Check sheet for the modelled part. Datum: model origin and axes. Units: mm. Face numbers are marked on the shaded views. A direction names the side the tool comes from. Give positions to 0.01 mm unless a question says otherwise; leave off trailing zeros. Loops run counter-clockwise (first coordinate to the right, second up) from the corner with the lowest first, then second, coordinate; pieces in that order, holes last. Notation, with made-up numbers: (12.5, 8.5) - (52.5, 8.5) arc R35 cw to (52.5, 41.5) - close; hole circle Ø10 at (-7, -14). An arc over 180 degrees is marked (long way). Use CSV: the item, a comma, the result in double quotes.
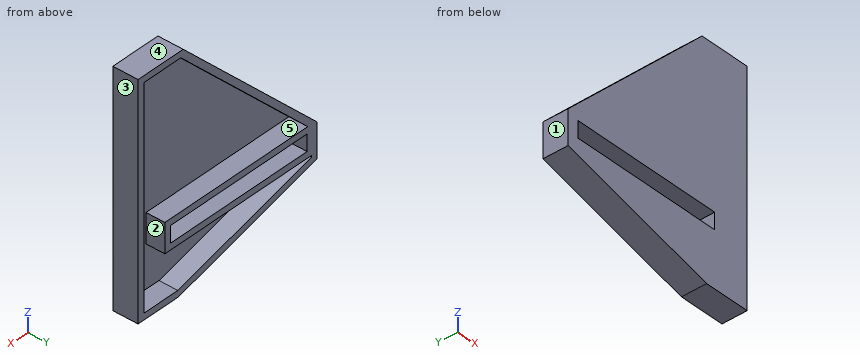
Autodesk Inventor part; units mm, degrees
ref_plane "YZ Plane" through (0, 0, 0) normal (1, 0, 0) x (0, 1, 0)
ref_plane "XZ Plane" through (0, 0, 0) normal (0, 1, 0) x (-1, 0, 0)
ref_plane "XY Plane" through (0, 0, 0) normal (0, 0, 1) x (1, 0, 0)
sketch "Sketch1" plane through (0, 0, 0) normal (0, 1, 0) x (-1, 0, 0)
  line L0 (0, 0) -> (90, 0)
  line L1 (90, 0) -> (90, -90)
  line L2 (90, -90) -> (0, -90)
  line L3 (0, -90) -> (0, 0)
  line L4 (0, 0) -> (90, 0)
  line L5 (90, 0) -> (90, -65)
  line L6 (90, -65) -> (0, -65)
  line L7 (0, -65) -> (0, 0)
  line L8 (14.5, -68.2385) -> (75.5, -68.2385)
  line L9 (75.5, -68.2385) -> (75.5, -61.7615)
  line L10 (75.5, -61.7615) -> (14.5, -61.7615)
  line L11 (14.5, -61.7615) -> (14.5, -68.2385)
  line L12 (14.5, -68.2385) -> (75.5, -61.7615) construction
  line L13 (75.5, -68.2385) -> (14.5, -61.7615) construction
  line L14 (14.5, -68.2385) -> (75.5, -68.2385) construction
  point P0 (45, -65)
  dimension "d16" = 90
  dimension "d17" = 90
  dimension "d18" = 90
  dimension "d19" = 65
  dimension "d20" = 61
  dimension "d21" = 0
  dimension "d22" = 6.477
extrude "Extrusion1" add sketch "Sketch1" along normal blind 10 contours L0 L1 L6 L9 L10 L11 L3 | L6 L11 L8 L9 L1 L2 L3
chamfer "Chamfer1" distance 69.85 angle 45 1 edges at (-90, 5, 0)
sketch "Sketch2" plane through (-90, 0, -69.85) normal (-1, 0, 0) x (0, 0, 1)
  line L0 (69.85, 10) -> (0, 10)
  line L1 (0, 10) -> (0, 0)
  line L2 (0, 0) -> (69.85, 0)
  line L3 (69.85, 0) -> (69.85, 10)
  line L4 (-20.15, 0) -> (0, 0)
  line L5 (0, 10) -> (0, 0)
  line L6 (-20.15, 10) -> (0, 10)
  line L7 (-7.8336, 10) -> (-20.15, 10)
  line L8 (-20.15, 10) -> (-20.15, 0)
  line L9 (-20.15, 0) -> (-7.8336, 0)
  line L10 (-7.8336, 0) -> (-7.8336, 10)
  line L11 (-20.15, 0) -> (-20.15, 10)
extrude "Extrusion2" cut sketch "Sketch2" against normal blind 10
chamfer "Chamfer3" distance 61.9125 angle 15 1 edges at (-80, 5, -90) measured on face at (-26.6667, 6.6667, -90)
shell "Shell1" thickness 2.54 removed faces 1 at (-36.7167, 10, -41.1743)
properties part number "Speaker Stand"
1. Release check for a two-part mould opening along X. For the marked faces 1, 2 and 3 record: released by +X, released by -X, zero draft, split by the parting line, or undercut.
Completed:
face 1,"released by -X"
face 2,"undercut"
face 3,"released by +X"
2. Sectioned sample at B-B, the plane x = -25.5. Record the boundary of the cut face in (y, z).
Completed:
outline,"(0, -88.01) - (10, -88.01) - (10, -85.38) - (2.54, -85.38) - (2.54, -70.78) - (10, -70.78) - (10, -68.24) - (0, -68.24) - close; (0, -61.76) - (10, -61.76) - (10, -59.22) - (2.54, -59.22) - (2.54, -8.94) - (10, -8.94) - (10, -5.35) - (0, -5.35) - close"
3. Set-up check for the marked faces 4 and 5: record each of +Z, -Z, +X, -X, +Y, -Y from which the full face is reachable in a straight line by a thin tool's end or side.
Completed:
face 4,"+Z, +X, -X, +Y, -Y"
face 5,"+Y"
4. Sectioned sample at D-D, the plane x = -6. Record the boundary of the cut face in (y, z), and give its area (3 significant figures).
Completed:
outline,"(0, -90) - (10, -90) - (10, -87.46) - (2.54, -87.46) - (2.54, -2.54) - (10, -2.54) - (10, 0) - (0, 0) - close"
area,"266 mm²"
5. Go/stop test with flat-tipped pins: pin 1 Ø22.5 at (x, z) = (-26.5, -35.5) entering from +Y; pin 2 Ø6 at (x, y) = (-60, 7.5) entering from -Z; pin 3 Ø2 at (x, y) = (-64, 2) entering from +Z. Record where each tip stops, or that it passes through.
Completed:
pin 1,"stops at y = 2.54"
pin 2,"stops at z = -79.57"
pin 3,"stops at z = -42.85"
6. Sectioned sample at C-C, the plane z = -18. Record the boundary of the cut face in (x, y).
Completed:
outline,"(-38.15, 0) - (0, 0) - (0, 10) - (-2.54, 10) - (-2.54, 2.54) - (-34.56, 2.54) - (-34.56, 10) - (-38.15, 10) - close"
7. Scan lines: line 1 along Z through (x, y) = (-15, 3.5); line 2 along Z through (x, y) = (-31.5, 4); line 3 along Y through (x, z) = (-71, -71). Record each from-to range of solid material in increasing order.
Completed:
line 1,"z = -90 to -87.46, -70.78 to -68.24, -61.76 to -59.22, -2.54 to 0"
line 2,"z = -86.41 to -83.78, -70.78 to -68.24, -61.76 to -59.22, -14.94 to -11.35"
line 3,"y = 0 to 2.54"
8. Sectioned sample at A-A, the plane y = 7.5. Record the boundary of the cut face in (x, z).
Completed:
outline,"(-80, -73.41) - (-18.09, -90) - (0, -90) - (0, 0) - (-20.15, 0) - (-80, -59.85) - close; hole (-77.46, -71.46) - (-17.75, -87.46) - (-2.54, -87.46) - (-2.54, -2.54) - (-19.1, -2.54) - (-75.78, -59.22) - (-11.96, -59.22) - (-11.96, -70.78) - (-77.46, -70.78) - close; hole (-75.5, -68.24) - (-14.5, -68.24) - (-14.5, -61.76) - (-75.5, -61.76) - close"
